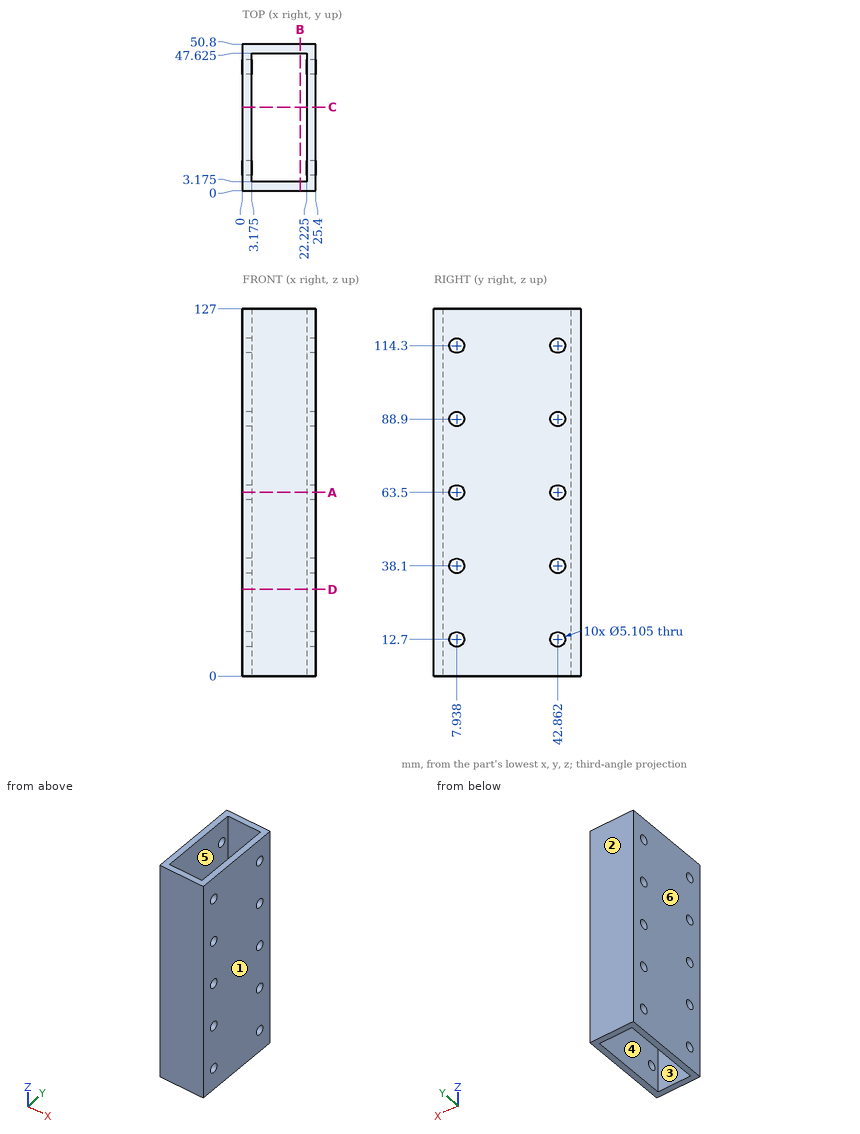
Design review of the part shown in the three views and the two pictorial views. Dimensions are in mm from the part's minimum x, y and z. A direction names the side the tool comes from. Round coordinates to 2 decimals unless told otherwise and drop trailing zeros. Write each loop counter-clockwise with the first axis right and the second up, starting at its lowest first coordinate (ties: lowest second). Pieces come first, ordered by that corner, then holes. Notation, with made-up numbers: (-20.75, 46) -> (-10.75, 46) arc R15 ccw to (-10.75, 50) -> close; hole circle Ø9 at (-4, -32). An arc over 180 degrees is marked (long way). Answer as a JSON object with one key per item and string values.
1. We need section B-B on x = 20. State the section outline as (y, z) points (1 decimal).
Results found:
{"outline": "(0, 0) -> (3.2, 0) -> (3.2, 127) -> (0, 127) -> close; (47.6, 0) -> (50.8, 0) -> (50.8, 127) -> (47.6, 127) -> close"}
2. Clearance check with a flat-ended pin moving along its axis: pin 1 (4 mm diameter, centred on y = 42.86, z = 63.5, fed in from -X). State where the tip first meets the part, or that it passes through.
Results found:
{"pin 1": "passes through"}
3. We need section C-C on y = 29. State the section outline as (x, z) points (1 decimal).
Results found:
{"outline": "(0, 0) -> (3.2, 0) -> (3.2, 127) -> (0, 127) -> close; (22.2, 0) -> (25.4, 0) -> (25.4, 127) -> (22.2, 127) -> close"}
4. We need section A-A on z = 63.5. State the section outline as (x, y) points (1 decimal).
Results found:
{"outline": "(0, 0) -> (25.4, 0) -> (25.4, 5.4) -> (22.2, 5.4) -> (22.2, 3.2) -> (3.2, 3.2) -> (3.2, 5.4) -> (0, 5.4) -> close; (0, 10.5) -> (3.2, 10.5) -> (3.2, 40.3) -> (0, 40.3) -> close; (0, 45.4) -> (3.2, 45.4) -> (3.2, 47.6) -> (22.2, 47.6) -> (22.2, 45.4) -> (25.4, 45.4) -> (25.4, 50.8) -> (0, 50.8) -> close; (22.2, 10.5) -> (25.4, 10.5) -> (25.4, 40.3) -> (22.2, 40.3) -> close"}
5. Machinability: for the marked faces 5 and 6, which of the approach directions +Z, -Z, +X, -X, +Y, -Y give a long, thin tool a straight path to every point of the face, cutting with its end or side? Answer none if there is none.
Results found:
{"face 5": "+Z, -Z", "face 6": "+Z, -Z, -X, +Y, -Y"}
6. To check wall thickness, follow line 1 along Y through (x, z) = (1.65, 63.5) (1 decimal); line 2 along X through (y, z) = (41.5, 96.5) (1 decimal); line 3 along Y through (x, z) = (12.5, 94.5) (1 decimal). State the ranges of each line that lie inside material, in increasing order.
Results found:
{"line 1": "y = 0 to 5.4, 10.5 to 40.3, 45.4 to 50.8", "line 2": "x = 0 to 3.2, 22.2 to 25.4", "line 3": "y = 0 to 3.2, 47.6 to 50.8"}
7. The part is to be moulded in two halves that separate along Y. For the marked faces 1, 2, 3 and 4, say which applies: pulls with the +Y half, pulls with the -Y half, needs draft (parallel to the pull), parting line crosses it, or undercut.
Results found:
{"face 1": "needs draft", "face 2": "pulls with the +Y half", "face 3": "undercut", "face 4": "undercut"}
8. We need section D-D on z = 30. State the section outline as (x, y) points (1 decimal).
Results found:
{"outline": "(0, 0) -> (25.4, 0) -> (25.4, 50.8) -> (0, 50.8) -> close; hole (3.2, 3.2) -> (22.2, 3.2) -> (22.2, 47.6) -> (3.2, 47.6) -> close"}
